Geometry check sheet. Reference: the model listing, model coordinates, mm. A direction names the side the tool comes from. Coordinates: 2 decimals unless noted, no trailing zeros. Write each loop counter-clockwise with the first axis right and the second up, starting at its lowest first coordinate (ties: lowest second). Pieces come first, ordered by that corner, then holes.
from build123d import *

# Parameters (mm, degrees)
F1_DEPTH = 1
F3_DEPTH = 25
F5_DEPTH = 25
F7_DEPTH = 1.5
F8_R     = 0.5


with BuildPart() as f1:
    # F0 (on Top) → F1 (new body)
    with BuildSketch(Plane.XY):
        with BuildLine():
            ThreePointArc((0, -3), (-1.7207293091, 2.4574561329), (2.8190778624, -1.02606043))
            Line((2.8190778624, -1.02606043), (4.6984631039, -1.7101007166))
            ThreePointArc((4.6984631039, -1.7101007166), (4.3301270189, 2.5), (0.8682408883, 4.9240387651))
            Line((0.8682408883, 4.9240387651), (0.6945927107, 3.939231012))
            ThreePointArc((0.6945927107, 3.939231012), (-2.2943057454, 3.2766081772), (-3.939231012, 0.6945927107))
            Line((-3.939231012, 0.6945927107), (-4.9240387651, 0.8682408883))
            ThreePointArc((-4.9240387651, 0.8682408883), (-3.8302222156, -3.2139380484), (0, -5))
            Line((0, -5), (0, -3))
        make_face()
        with BuildLine():
            Line((0.6945927107, 3.939231012), (0.8682408883, 4.9240387651))
            ThreePointArc((0.8682408883, 4.9240387651), (-2.8678821818, 4.0957602214), (-4.9240387651, 0.8682408883))
            Line((-4.9240387651, 0.8682408883), (-3.939231012, 0.6945927107))
            ThreePointArc((-3.939231012, 0.6945927107), (-2.2943057454, 3.2766081772), (0.6945927107, 3.939231012))
        make_face()
    extrude(amount=F1_DEPTH)

    # F2 (on face) → F3 (cut)
    with BuildSketch(Plane(origin=(0, 0, 0), x_dir=(0.9396926208, -0.3420201433, 0), z_dir=(-0.3420201433, -0.9396926208, 0))):
        Polygon((3, 0.6489407005), (5, 0), (5, 1), (3, 1), align=None)
        Polygon((1.9180543022, 1), (3, 0.6489407005), (3, 1), align=None)
    extrude(amount=-F3_DEPTH, mode=Mode.SUBTRACT)

    # F4 (on face) → F5 (cut)
    with BuildSketch(Plane.YZ):
        Polygon((-5, 1), (-5, 0), (-1.91805, 1), align=None)
    extrude(amount=-F5_DEPTH, mode=Mode.SUBTRACT)

    # F6 (on face) → F7 (join)
    with BuildSketch(Plane.XY.offset(1)):
        with BuildLine():
            ThreePointArc((-3.7702121506, 1.3722449997), (-2.3012895939, 3.2865821464), (0, 4.0121759682))
            Line((0, 4.0121759682), (0.1736481777, 4.9969837212))
            ThreePointArc((0.1736481777, 4.9969837212), (-2.8678821818, 4.0957602214), (-4.7550199037, 1.5458931774))
            Line((-4.7550199037, 1.5458931774), (-3.7702121506, 1.3722449997))
        make_face()
    extrude(amount=F7_DEPTH)

    # F8
    f8_edges = [f1.edges().sort_by_distance(p)[0] for p in [
        (-4.262616, 1.459069, 2.5),
        (0.086824, 4.50458, 2.5),
        (-2.867882, 4.09576, 2.5),
    ]]
    fillet(f8_edges, radius=F8_R)


solid = f1.part
1. Gauge pin test, flat ends, axial feed: pin 1 Ø5 at (x, y) = (2.5, -3) entering from +Z; pin 2 Ø1 at (x, z) = (2.5, 1) entering from +Y. Record the tip position at first contact, or that the pin passes through.
Computed values:
pin 1: stops at z = 0.66
pin 2: stops at y = 4.58
2. Sectioned sample at A-A, the plane y = 1.25. Record the boundary of the cut face in (x, z), and give its area (3 significant figures).
Computed values:
outline: (-4.84, 0) - (-2.73, 0) - (-2.73, 1) - (-4.84, 1) - close; (2.73, 0) - (4.84, 0) - (4.84, 0.28) - (2.73, 0.93) - close
area: 3.40 mm2
3. Sectioned sample at B-B, the plane y = 0. Record the boundary of the cut face in (x, z), and give its area (3 significant figures).
Computed values:
outline: (-5, 0) - (-3, 0) - (-3, 1) - (-5, 1) - close; (3, 0) - (5, 0) - (5, 0.1) - (3, 0.71) - close
area: 2.81 mm2
4. Access from +Z, -Z, +X, -X, +Y, -Y to the whole of each face (thin tool, end or side, straight path). Record for faces 4 (the flat face through (-4.27, 1.46, 1.49)), 5 (the flat face through (0.086, 4.498, 1.493)), 6 (the flat face through (-2.3, 2.3, 0)).
Computed values:
face 4: +Z, -X, -Y
face 5: +Z, +X, -Y
face 6: -Z, +X, -X, +Y, -Y
5. Thickness scan on line 1 along Z through (x, y) = (-3.75, -3); line 2 along X through (y, z) = (0, 0.75); line 3 along Z through (x, y) = (-4.5, -0.25). Record the ranges inside material, lowest first.
Computed values:
line 1: z = 0 to 0.65
line 2: x = -5 to -3
line 3: z = 0 to 1
6. Sectioned sample at C-C, the plane z = 1.15. Record the boundary of the cut face in (x, y), and give its area (3 significant figures).
Computed values:
outline: (-4.76, 1.55) - (-3.77, 1.37) arc R4.01 cw to (0, 4.01) - (0.17, 5) arc R5 ccw to start
area: 5.61 mm2
7. Sectioned sample at D-D, the plane x = 0.5. Record the boundary of the cut face in (y, z).
Computed values:
outline: (2.96, 0) - (4.97, 0) - (4.97, 1) - (2.96, 1) - close
8. Draft check along X on faces 1 (the cylindrical face through (-1.8, 2.4, 0.5)), 2 (the flat face through (-1.763, -3.481, 0.493)), 3 (the cylindrical face through (-2.329, 3.267, 1.74)). Enter one of: released by +X, released by -X, zero draft, split by the parting line, or undercut.
Computed values:
face 1: undercut
face 2: zero draft
face 3: released by +X
